```python
from build123d import *

# Parameters (mm, degrees)
BOSS_EXTRUDE1_DEPTH = 2.5
SKETCH2_R           = 1.625
BOSS_EXTRUDE2_DEPTH = 5.5
CHAMFER1_SIZE       = 0.5
FILLET2_R           = 2


with BuildPart() as part:
    # Sketch1 → Boss-Extrude1 (new, symmetric)
    with BuildSketch(Plane(origin=(0, 0, 0), x_dir=(1, 0, 0), z_dir=(0, 1, 0))):
        with BuildLine():
            Line((0, 0), (31.692840332, 0))
            ThreePointArc((31.692840332, 0), (31.114494888, 2.721592177), (29.479411171, 4.972824878))
            Line((29.479411171, 4.972824878), (23.85490024, 10.039260498))
            ThreePointArc((23.85490024, 10.039260498), (13.799067859, 24.384002459), (11.023460035, 41.68103654))
            ThreePointArc((11.023460035, 41.68103654), (10.905516567, 42.089144278), (10.553169202, 42.326449823))
            Line((10.553169202, 42.326449823), (0, 0))
        make_face()
    extrude(amount=BOSS_EXTRUDE1_DEPTH, both=True)

    # Sketch2 → Boss-Extrude2 (add)
    with BuildSketch(Plane(origin=(0, 0, 0), x_dir=(-0.24192189559966498, 0, 0.9702957262759973), z_dir=(-0.9702957262759971, 0, -0.24192189559966495))):
        with Locations(Location((-5, 0, 0), (0, 0, 180))):
            Circle(SKETCH2_R)
    extrude(amount=BOSS_EXTRUDE2_DEPTH)

    # Chamfer1
    chamfer1_edges = [part.edges().sort_by_distance(p)[0] for p in [
        (-4.520140097, 0, -4.605318502),
    ]]
    chamfer(chamfer1_edges, length=CHAMFER1_SIZE)

    # Sketch3 → Cut-Revolve4 (revolve, cut)
    with BuildSketch(Plane(origin=(0, 0, 0), x_dir=(1, 0, 0), z_dir=(0, 1, 0))):
        with BuildLine():
            Line((0.816486398, 3.274748076), (0.707621545, 2.838114999))
            ThreePointArc((0.707621545, 2.838114999), (0.73826383, 2.905034263), (0.791037406, 2.956338134))
            Line((0.791037406, 2.956338134), (0.863180576, 3.004248082))
            ThreePointArc((0.863180576, 3.004248082), (0.928011981, 3.154719604), (0.816486398, 3.274748076))
        make_face()
    revolve(axis=Axis((-4.382099311, 0, -6.245648216), (0.9702957262759973, 0, 0.2419218955996649)), mode=Mode.SUBTRACT)

    # Fillet2
    # the kernel refuses this fillet: 2 mm, written as the material it takes off along each edge
    with BuildSketch(Plane(origin=(25, -2.5, 0), x_dir=(0.7336270149477808, 0, 0.6795523548180881), z_dir=(-0.6795523548180881, 0, 0.7336270149477808))) as fillet2_piece_1:
        with BuildLine():
            CenterArc((6.692840332 - FILLET2_R, FILLET2_R), FILLET2_R, 270, 90)
            Line((6.692840332, FILLET2_R), (6.692840332, 0))
            Line((6.692840332, 0), (6.692840332 - FILLET2_R, 0))
        make_face()
    revolve(axis=Axis((25, -2.5, 0), (0, 1, 0)), revolution_arc=90.796842199, mode=Mode.SUBTRACT)
    with BuildSketch(Plane(origin=(29.479411171, -2.5, -4.972824878), x_dir=(-0.6692840332038654, 0, 0.7430066506420836), z_dir=(-0.7430066506420837, 0, -0.6692840332038654))) as fillet2_piece_2:
        with BuildLine():
            CenterArc((FILLET2_R, FILLET2_R), FILLET2_R, 180, 90)
            Line((0, FILLET2_R), (0, 0))
            Line((0, 0), (FILLET2_R, 0))
        make_face()
    extrude(amount=7.569933494, mode=Mode.SUBTRACT)
    with BuildSketch(Plane(origin=(50, -2.5, -39.064281325), x_dir=(-0.6692840332038644, 0, 0.7430066506420845), z_dir=(0.7430066506420845, 0, 0.6692840332038644))) as fillet2_piece_3:
        with BuildLine():
            CenterArc((39.064281325 + FILLET2_R, -FILLET2_R), FILLET2_R, 90, 90)
            Line((39.064281325, -FILLET2_R), (39.064281325, 0))
            Line((39.064281325, 0), (39.064281325 + FILLET2_R, 0))
        make_face()
    revolve(axis=Axis((50, -2.5, -39.064281325), (0, -1, 0)), revolution_arc=59.163556195, mode=Mode.SUBTRACT)


solid = part.part
```
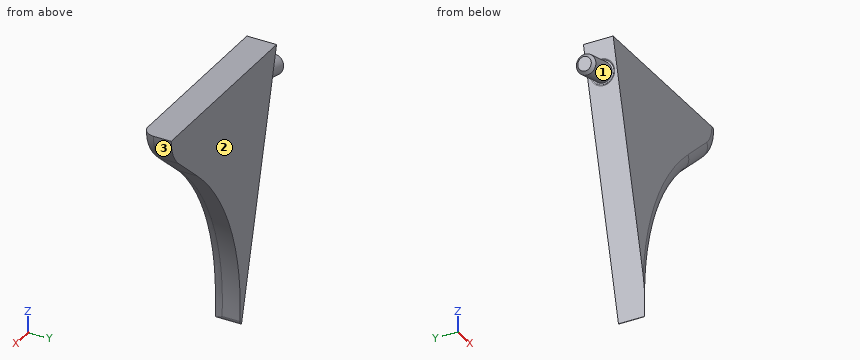
The model under review builds one solid part; all positions refer to its coordinate system, in mm. Face numbers are marked on the shaded views. Coordinates: 2 decimals unless noted, no trailing zeros. Write each loop counter-clockwise with the first axis right and the second up, starting at its lowest first coordinate (ties: lowest second). Pieces come first, ordered by that corner, then holes.
1) To check wall thickness, follow probe 1 along X at (y, z) = (0.45, -29.5); probe 2 along X at (y, z) = (-0.95, -10); probe 3 along Z at (x, y) = (24, 0.35). State the ranges of each line that lie inside material, in increasing order.
2) Clearance check with flat-ended pins moving along their axes: pin 1 Ø1 at (y, z) = (-1, -30.5) entering from -X; pin 2 Ø1.5 at (y, z) = (1, -29) entering from +X; pin 3 Ø1 at (y, z) = (2, -27.5) entering from -X. State where each tip first meets the part, or that it passes through.
3) We need section A-A on x = 3.5. State the section outline as (y, z) points, then the cut area to 3 significant figures.
4) The part is to be moulded in two halves that separate along X. For the marked faces 1, 2 and 3, say which applies: pulls with the +X half, pulls with the -X half, needs draft (parallel to the pull), parting line crosses it, or undercut.
Answer list:
1. probe 1: x = 7.36 to 12.12
1. probe 2: x = 2.49 to 23.82
1. probe 3: z = -9.91 to 0
2. pin 1: stops at x = 7.48
2. pin 2: stops at x = 12.46
2. pin 3: stops at x = 6.73
3. outline: (-2.5, -14.04) - (2.5, -14.04) - (2.5, 0) - (-2.5, 0) - close
3. area: 70.2 mm2
4. face 1: undercut
4. face 2: needs draft
4. face 3: pulls with the +X half
